from build123d import *

# Parameters (mm, degrees)
SKETCH_1_W      = 22
SKETCH_1_H      = 54
SKETCH_1_W_2    = 18
SKETCH_1_H_2    = 50
EXTRUDE_1_DEPTH = 100
SKETCH_2_W      = 22
SKETCH_2_H      = 54
EXTRUDE_2_DEPTH = 0.1
SKETCH_3_R      = 2
EXTRUDE_3_DEPTH = 22


with BuildPart() as part:
    # 草图1 → 凸台-拉伸1 (new body)
    with BuildSketch(Plane(origin=(0, 0, 0), x_dir=(1, 0, 0), z_dir=(0, 1, 0))):
        Rectangle(SKETCH_1_W, SKETCH_1_H)
        Rectangle(SKETCH_1_W_2, SKETCH_1_H_2, mode=Mode.SUBTRACT)
    extrude(amount=EXTRUDE_1_DEPTH)

    # 草图2 → 凸台-拉伸2 (add)
    with BuildSketch(Plane(origin=(0, 100, 0), x_dir=(1, 0, 0), z_dir=(0, 1, 0))):
        Rectangle(SKETCH_2_W, SKETCH_2_H)
    extrude(amount=EXTRUDE_2_DEPTH)

    # 草图3 → 凸台-拉伸3 (add)
    with BuildSketch(Plane.ZY.offset(11)):
        with Locations((0, 64.062893105)):
            Circle(SKETCH_3_R)
        with Locations((0, 53.062893105)):
            Circle(SKETCH_3_R)
    extrude(amount=-EXTRUDE_3_DEPTH)


solid = part.part
Work out the finished part from the listing and answer in its coordinate system (mm). A direction names the side the tool comes from. Coordinates: 2 decimals unless noted, no trailing zeros. Write each loop counter-clockwise with the first axis right and the second up, starting at its lowest first coordinate (ties: lowest second). Pieces come first, ordered by that corner, then holes. Notation, with made-up numbers: M 83.25,-21 L 99.25,-21 A23 ccw 99.25,14 Z; hole C 65.25,65 d7. An arc over 180 degrees is marked long. Use one line per item in the form item = value. Start each with the question number.
1. Straight lines are drawn through the part: probe 1 along Z at (x, y) = (-8.75, 6.5); probe 2 along X at (y, z) = (35.5, -15.5); probe 3 along Z at (x, y) = (3.5, 51.5). For each, find the intervals that lie inside material, in ascending order. Write a range as from..to.
2. The part is cut by section D-D (z = 0). Give the vertices of the cut face in (x, y).
3. The part is cut by section A-A (y = 30.5). Give the vertices of the cut face in (x, z), plus the area to 3 significant figures.
4. The part is cut by section B-B (z = 19). Give the vertices of the cut face in (x, y), plus the area to 3 significant figures.
5. The mould has two halves that part along Y. Classify faces 1 (the face through (-0.126, 51.289, 0.923)), 2 (the face through (-0.126, 62.289, 0.923)), 3 (the face through (-10, 0, -8)), 4 (the face through (0, 49, 25)): released by +Y, released by -Y, zero draft, split by the parting line, or undercut.
6. Each of these flat-tipped pins is pushed along its axis until it touches: P1, Ø9, axis at x = 0, z = 8, coming from the -Y side; P2, Ø2, axis at x = -5.5, z = 0.5, coming from the -Y side. Where does it stop, or does it pass through?
7. A tool of negligible diameter and unlimited length cuts with its end or side. For faces 5 (the face through (0, 49, -27)), 6 (the face through (0, 49, -25)), from which of +Z, -Z, +X, -X, +Y, -Y can it reach the whole face along a straight path? Write none if from no direction.
8. The part is cut by section C-C (x = 6.75). Give the vertices of the cut face in (y, z).
Evaluation:
q1.probe_1 = -27..-25, 25..27
q1.probe_2 = -11..-9, 9..11
q1.probe_3 = -27..-25, -1.25..1.25, 25..27
q2.outline = M -11,0 L -9,0 L -9,51.06 L 9,51.06 L 9,0 L 11,0 L 11,100.1 L -11,100.1 Z; hole M -9,55.06 L 9,55.06 L 9,62.06 L -9,62.06 Z; hole M -9,66.06 L 9,66.06 L 9,100 L -9,100 Z
q3.outline = M -11,-27 L 11,-27 L 11,27 L -11,27 Z; hole M -9,-25 L 9,-25 L 9,25 L -9,25 Z
q3.area = 288 mm^2
q4.outline = M -11,0 L -9,0 L -9,100 L 9,100 L 9,0 L 11,0 L 11,100.1 L -11,100.1 Z
q4.area = 402 mm^2
q5.face_1 = undercut
q5.face_2 = undercut
q5.face_3 = released by -Y
q5.face_4 = zero draft
q6.P1 = 100
q6.P2 = 51.06
q7.face_5 = -Z, +X, -X, +Y, -Y
q7.face_6 = -Y
q8.outline = M 0,-27 L 100.1,-27 L 100.1,27 L 0,27 L 0,25 L 100,25 L 100,-25 L 0,-25 Z; C 53.06,0 d4; C 64.06,0 d4
